from build123d import *

# Parameters (mm, degrees)
SKETCH1_R           = 45.72
BOSS_EXTRUDE1_DEPTH = 5
SKETCH2_R           = 9.6
SKETCH2_R_2         = 4.5
CUT_EXTRUDE1_DEPTH  = 4
SKETCH3_R           = 4.5
CUT_EXTRUDE2_DEPTH  = 65.781454136
FILLET1_R           = 4
FILLET2_R           = 0.5


with BuildPart() as part:
    # Sketch1 → Boss-Extrude1 (new body)
    with BuildSketch(Plane(origin=(0, 0, 0), x_dir=(1, 0, 0), z_dir=(0, 1, 0))):
        with Locations(Location((0, 0, 0), (0, 0, 270))):
            Circle(SKETCH1_R)
    extrude(amount=BOSS_EXTRUDE1_DEPTH)

    # Sketch2 → Cut-Extrude1 (cut)
    # profile 1 of 2: a face of its own
    with BuildSketch(Plane(origin=(0, 5, 0), x_dir=(1, 0, 0), z_dir=(0, 1, 0))):
        with Locations(Location((0, 0, 0), (0, 0, 270))):
            Circle(SKETCH2_R)
        Circle(SKETCH2_R_2, mode=Mode.SUBTRACT)
    # profile 2 of 2: a face of its own
    with BuildSketch(Plane(origin=(0, 5, 0), x_dir=(1, 0, 0), z_dir=(0, 1, 0))):
        Circle(SKETCH2_R_2)
    extrude(amount=-CUT_EXTRUDE1_DEPTH, mode=Mode.SUBTRACT)

    # Sketch3 → Cut-Extrude2 (cut, through all)
    with BuildSketch(Plane(origin=(0, 1, 0), x_dir=(1, 0, 0), z_dir=(0, 1, 0))):
        with Locations(Location((0, 0, 0), (0, 0, 270))):
            Circle(SKETCH3_R)
    extrude(amount=-CUT_EXTRUDE2_DEPTH, mode=Mode.SUBTRACT)

    # Fillet1
    fillet1_edges = [part.edges().sort_by_distance(p)[0] for p in [
        (0, 5, -45.72),
    ]]
    fillet(fillet1_edges, radius=FILLET1_R)

    # Fillet2
    fillet2_edges = [part.edges().sort_by_distance(p)[0] for p in [
        (0, 5, -9.6),
    ]]
    fillet(fillet2_edges, radius=FILLET2_R)


solid = part.part
Build history of the part. All positions in model axes, mm. A direction names the side the tool comes from. Round coordinates to 2 decimals unless told otherwise and drop trailing zeros. Loops run counter-clockwise (first coordinate to the right, second up) from the corner with the lowest first, then second, coordinate; pieces in that order, holes last. Notation, with made-up numbers: (55, -3) -> (64, -3) arc R20 ccw to (64, 10) -> close; hole circle Ø1 at (66, -34.5). An arc over 180 degrees is marked (long way). One line per item, written item: value. Start each with the question number.
Q1. Two-plate mould, pull along Z, no slides. Class faces 3 (the face through (2.3, 1, 4.1)), 4 (the face through (-10, 0, -1)), 5 (the face through (45.33, 0.49, -5.95)): released by +Z, released by -Z, zero draft, split by the parting line, or undercut.
Q2. 3-axis set-ups, long thin cutter, end or side, ignore diameter. For faces 1 (the face through (1.352, 0.507, 4.292)), 2 (the face through (8.095, 2.774, 5.161)): which of +Z, -Z, +X, -X, +Y, -Y reach the whole face in a straight line?
Q3. Cut at B-B on x = 0. List the corners of the cut face in (y, z), plus the area to 3 significant figures.
Q4. Cut at A-A on z = 0. List the corners of the cut face in (x, y), plus the area to 3 significant figures.
Q5. Cut at C-C on y = 2.75. List the corners of the cut face in (x, z).
Q6. Probe line 1 along X through (y, z) = (0.75, 0); line 2 along X through (y, z) = (2.4, 0); line 3 along Y through (x, z) = (5.5, -1.5). List the from-to ranges inside material, lowest first.
Q7. Drop flat-ended pins along their axis: pin 1 Ø3 at (x, z) = (-8.5, 12.5) entering from -Y; pin 2 Ø1 at (y, z) = (2, -30) entering from -X; pin 3 Ø7 at (x, z) = (0, 0) entering from -Y; pin 4 Ø3 at (y, z) = (0.5, -29) entering from -X. Give the stop position or say it passes through.
Computed:
1. face 3: undercut
1. face 4: zero draft
1. face 5: split by the parting line
2. face 1: +Y, -Y
2. face 2: +Y
3. outline: (0, -45.72) -> (1, -45.72) arc R4 ccw to (5, -41.72) -> (5, -10.1) arc R0.5 ccw to (4.5, -9.6) -> (1, -9.6) -> (1, -4.5) -> (0, -4.5) -> close; (0, 4.5) -> (1, 4.5) -> (1, 9.6) -> (4.5, 9.6) arc R0.5 ccw to (5, 10.1) -> (5, 41.72) arc R4 ccw to (1, 45.72) -> (0, 45.72) -> close
3. area: 364 mm²
4. outline: (-45.72, 0) -> (-4.5, 0) -> (-4.5, 1) -> (-9.6, 1) -> (-9.6, 4.5) arc R0.5 ccw to (-10.1, 5) -> (-41.72, 5) arc R4 ccw to (-45.72, 1) -> close; (4.5, 0) -> (45.72, 0) -> (45.72, 1) arc R4 ccw to (41.72, 5) -> (10.1, 5) arc R0.5 ccw to (9.6, 4.5) -> (9.6, 1) -> (4.5, 1) -> close
4. area: 364 mm²
5. outline: circle Ø90.63 at (0, 0); hole circle Ø19.2 at (0, 0)
6. line 1: -45.72 to -4.5, 4.5 to 45.72
6. line 2: -45.47 to -9.6, 9.6 to 45.47
6. line 3: 0 to 1
7. pin 1: y = 0
7. pin 2: x = -34.79
7. pin 3: through
7. pin 4: x = -36.52
